```python
from build123d import *

# Parameters (mm, degrees)
SKETCH1_R           = 1.65
BOSS_EXTRUDE1_DEPTH = 2
SKETCH3_W           = 18
SKETCH3_H           = 12
BOSS_EXTRUDE3_DEPTH = 2
SKETCH3_3_W         = 20
SKETCH3_3_H         = 3
SKETCH3_3_H_2       = 6
BOSS_EXTRUDE4_DEPTH = 9.5
FILLET1_R           = 1
FILLET2_R           = 3
FILLET3_R           = 1


with BuildPart() as part:
    # Sketch1 → Boss-Extrude1 (new body)
    with BuildSketch(Plane(origin=(0, 0, 0), x_dir=(1, 0, 0), z_dir=(0, 1, 0))):
        with BuildLine():
            Line((-26, 42), (0, 42))
            Line((0, 42), (0, 0))
            Line((0, 0), (-26, 0))
            Line((-26, 0), (-26, 9.438307568))
            ThreePointArc((-26, 9.438307568), (-27.419949552, 12.327836077), (-30.575, 12.969153784))
            ThreePointArc((-30.575, 12.969153784), (-35.15, 16.5), (-30.575, 20.030846216))
            ThreePointArc((-30.575, 20.030846216), (-27.419949552, 20.672163923), (-26, 23.561692432))
            Line((-26, 23.561692432), (-26, 42))
        make_face()
        with Locations(Location((-31.5, 16.5, 0), (0, 0, 270))):
            Circle(SKETCH1_R, mode=Mode.SUBTRACT)
    extrude(amount=BOSS_EXTRUDE1_DEPTH)

    # Sketch3 → Boss-Extrude3 (add)
    with BuildSketch(Plane(origin=(0, 0, 0), x_dir=(1, 0, 0), z_dir=(0, 1, 0))):
        with Locations((-15, 16.5)):
            Rectangle(SKETCH3_W, SKETCH3_H)
    extrude(amount=-BOSS_EXTRUDE3_DEPTH)

    # Sketch3<3> → Boss-Extrude4 (add)
    with BuildSketch(Plane(origin=(0, 0, 0), x_dir=(1, 0, 0), z_dir=(0, 1, 0))):
        with Locations((-14.5, 3.75)):
            Rectangle(SKETCH3_3_W, SKETCH3_3_H)
        with Locations((-14.5, 35.5)):
            Rectangle(SKETCH3_3_W, SKETCH3_3_H_2)
    extrude(amount=-BOSS_EXTRUDE4_DEPTH)

    # Fillet1
    fillet1_edges = [part.edges().sort_by_distance(p)[0] for p in [
        (-24.5, 0, -3.75),
        (-4.5, 0, -3.75),
        (-14.5, 0, -2.25),
        (-14.5, 0, -38.5),
        (-4.5, 0, -35.5),
        (-24.5, 0, -35.5),
    ]]
    fillet(fillet1_edges, radius=FILLET1_R)

    # Fillet2
    fillet2_edges = [part.edges().sort_by_distance(p)[0] for p in [
        (-6, -1, -10.5),
        (-24, -1, -10.5),
        (-24, -1, -22.5),
        (-6, -1, -22.5),
    ]]
    fillet(fillet2_edges, radius=FILLET2_R)

    # Fillet3
    fillet3_edges = [part.edges().sort_by_distance(p)[0] for p in [
        (-26, 1, -42),
        (0, 1, -42),
        (0, 1, 0),
        (-26, 1, 0),
    ]]
    fillet(fillet3_edges, radius=FILLET3_R)


solid = part.part
```
CAD build for the part. Positions are in the model's coordinates, mm. A direction names the side the tool comes from. Coordinates: 2 decimals unless noted, no trailing zeros. Order: outer loops, then holes, each group sorted by start corner. A loop starts at its lowest first (then second) coordinate and runs counter-clockwise, first axis right, second up.
(1) Which spindle directions (+Z, -Z, +X, -X, +Y, -Y) get a long thin tool onto all of the face, cutting with end or side? Do faces 1 (the face through (-15, -5, -38.5)), 2 (the face through (-4.5, -5, -4)), 3 (the face through (-23.1, -1.01, -11.36)), 4 (the face through (-26, 1, -5)). Say none if no direction does.
Solution:
face 1: -Z, +X, -X, -Y
face 2: +Z, -Z, +X, -Y
face 3: -X, -Y
face 4: +Z, -X, +Y, -Y
(2) Drill centre lines: L1, parallel to Z at x = -13, y = -1.25; L2, parallel to Z at x = -18.5, y = -7.5; L3, parallel to Z at x = -22.5, y = -1.75. Where is each one in solid material? Low to high.
Solution:
L1: z = -38.5 to -32.5, -22.5 to -10.5, -5.25 to -2.25
L2: z = -38.5 to -32.5, -5.25 to -2.25
L3: z = -38.5 to -32.5, -22.1 to -10.9, -5.25 to -2.25
(3) Saw through at C-C, the plane x = -31.5. Write the cut outline in (y, z), and give its area (3 significant figures).
Solution:
outline: (0, -20.15) - (2, -20.15) - (2, -18.15) - (0, -18.15) - close; (0, -14.85) - (2, -14.85) - (2, -12.85) - (0, -12.85) - close
area: 8.00 mm2
(4) Mould opens along Z. For faces 5 (the face through (-15, -1, -10.5)), 6 (the face through (-14.346, -0.285, -38.801)), 7 (the face through (-4.199, -0.285, -36.049)) say: released by +Z, released by -Z, zero draft, split by the parting line, or undercut.
Solution:
face 5: undercut
face 6: released by -Z
face 7: zero draft
(5) Saw through at B-B, the plane z = -16.5. Write the cut outline in (x, y).
Solution:
outline: (-35.15, 0) - (-33.15, 0) - (-33.15, 2) - (-35.15, 2) - close; (-29.85, 0) - (-24, 0) - (-24, -2) - (-6, -2) - (-6, 0) - (0, 0) - (0, 2) - (-29.85, 2) - close
(6) Saw through at D-D, the plane z = -3.5. Write the cut outline in (x, y), and give its area (3 significant figures).
Solution:
outline: (-26, 0) - (-25.5, 0) arc R1 cw to (-24.5, -1) - (-24.5, -9.5) - (-4.5, -9.5) - (-4.5, -1) arc R1 cw to (-3.5, 0) - (0, 0) - (0, 2) - (-26, 2) - close
area: 242 mm2
(7) Pin check, flat tips, straight feed: pin 1 Ø2 at (y, z) = (-4.5, -13) entering from -X; pin 2 Ø5 at (x, y) = (-16, -7) entering from -Z; pin 3 Ø1.6 at (y, z) = (0.5, -3.5) entering from -X; pin 4 Ø6 at (x, z) = (-15, -16) entering from -Y. Stop position of each tip, or through.
Solution:
pin 1: passes through
pin 2: stops at z = -38.5
pin 3: stops at x = -26
pin 4: stops at y = -2
(8) Saw through at A-A, the plane y = -3.25. Write the cut outline in (x, z).
Solution:
outline: (-24.5, -38.5) - (-4.5, -38.5) - (-4.5, -32.5) - (-24.5, -32.5) - close; (-24.5, -5.25) - (-4.5, -5.25) - (-4.5, -2.25) - (-24.5, -2.25) - close
